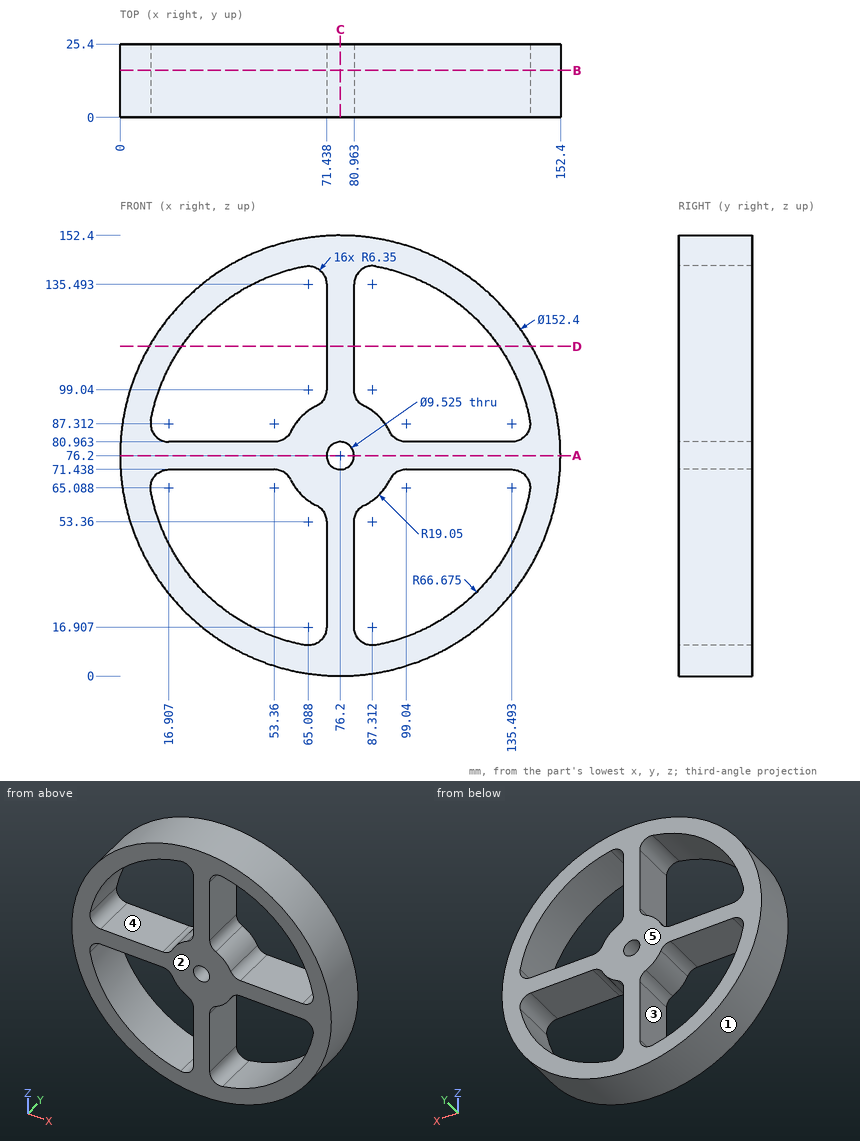
Geometry check sheet. Reference: drawing and pictorial views, mm from the part's lowest x, y, z. A direction names the side the tool comes from. Round coordinates to 2 decimals unless told otherwise and drop trailing zeros. Order: outer loops, then holes, each group sorted by start corner. A loop starts at its lowest first (then second) coordinate and runs counter-clockwise, first axis right, second up.
Q1. Scan lines: L1, parallel to Z at x = 76.2, y = 10.5; L2, parallel to X at y = 16.75, z = 115 (1 decimal); L3, parallel to X at y = 21.25, z = 113 (1 decimal). Record each from-to range of solid material in increasing order.
Filled sheet:
L1: z = 0 to 71.44, 80.96 to 152.4
L2: x = 10.6 to 22, 71.4 to 81, 130.4 to 141.8
L3: x = 9.5 to 20.6, 71.4 to 81, 131.8 to 142.9
Q2. Cross-section at D-D, the plane z = 114. Enter the section's corners in (x, y) (1 decimal), plus the area to 3 significant figures.
Filled sheet:
outline: (10, 0) - (21.3, 0) - (21.3, 25.4) - (10, 25.4) - close; (71.4, 0) - (81, 0) - (81, 25.4) - (71.4, 25.4) - close; (131.1, 0) - (142.4, 0) - (142.4, 25.4) - (131.1, 25.4) - close
area: 813 mm2
Q3. Cross-section at B-B, the plane y = 16.25. Give the number of separate pieces and of enclosed holes in the cut face.
Filled sheet:
separate pieces: 1
enclosed holes: 5
Q4. Set-up check for the marked faces 4 and 5: record each of +Z, -Z, +X, -X, +Y, -Y from which the full face is reachable in a straight line by a thin tool's end or side.
Filled sheet:
face 4: +Y, -Y
face 5: +Z, -Z, +X, -X, +Y
Q5. Cross-section at C-C, the plane x = 76.2. Enter the section's corners in (y, z), plus the area to 3 significant figures.
Filled sheet:
outline: (0, 0) - (25.4, 0) - (25.4, 71.44) - (0, 71.44) - close; (0, 80.96) - (25.4, 80.96) - (25.4, 152.4) - (0, 152.4) - close
area: 3,630 mm2
Q6. Depth check by flat-ended pin: P1, Ø7.5, axis at x = 118.5, y = 16.5, coming from the -Z side; P2, Ø7.5, axis at x = 41, y = 13, coming from the -Z side; P3, Ø7.5, axis at y = 17, z = 32.5, coming from the -X side; P4, Ø12, axis at x = 105.5, z = 122.5, coming from the +Y side. Enter the tip coordinate at first touch or a pass-through.
Filled sheet:
P1: stops at z = 10.47
P2: stops at z = 6.79
P3: stops at x = 11.31
P4: passes through
Q7. Cross-section at A-A, the plane z = 76.2. Enter the section's corners in (x, y), plus the area to 3 significant figures.
Filled sheet:
outline: (0, 0) - (71.44, 0) - (71.44, 25.4) - (0, 25.4) - close; (80.96, 0) - (152.4, 0) - (152.4, 25.4) - (80.96, 25.4) - close
area: 3,630 mm2
Q8. Draft check along X on the marked faces 1, 2 and 3. Enter one of: pulls with the +X half, pulls with the -X half, needs draft (parallel to the pull), parting line crosses it, or undercut.
Filled sheet:
face 1: parting line crosses it
face 2: needs draft
face 3: undercut
